For this review, take the finished solid that the model builds, in its own axes (mm). A direction names the side the tool comes from. Round coordinates to 2 decimals unless told otherwise and drop trailing zeros. Order: outer loops, then holes, each group sorted by start corner. A loop starts at its lowest first (then second) coordinate and runs counter-clockwise, first axis right, second up. Notation, with made-up numbers: M 14.25,50.5 L 24.25,50.5 A31 cw 24.25,74.5 Z; hole C -28,73 d8. An arc over 180 degrees is marked long. Answer as a JSON object with one key per item and string values.
from build123d import *

# Parameters (mm, degrees)
SKETCH1_W                        = 203.2
SKETCH1_H                        = 50.8
BOSS_EXTRUDE1_DEPTH              = 1
SKETCH1_3_R                      = 6.477
BOSS_EXTRUDE2_DEPTH              = 2.54
SKETCH2_W                        = 4.9022
SKETCH2_H                        = 3.54
F_3_8_CLEARANCE_HOLE1_AT_2_COUNT = 2
F_3_8_CLEARANCE_HOLE1_AT_2_PITCH = 69.85
F_3_8_CLEARANCE_HOLE1_AT_3_COUNT = 2
F_3_8_CLEARANCE_HOLE1_AT_3_PITCH = 139.7
F_3_8_CLEARANCE_HOLE1_AT_4_COUNT = 2
F_3_8_CLEARANCE_HOLE1_AT_4_PITCH = 69.85
FILLET1_R                        = 12.7


with BuildPart() as part:
    # Sketch1 → Boss-Extrude1 (new body)
    with BuildSketch(Plane.XY):
        with Locations((-9.525, 0)):
            Rectangle(SKETCH1_W, SKETCH1_H)
    extrude(amount=BOSS_EXTRUDE1_DEPTH)

    # Sketch1<3> → Boss-Extrude2 (add)
    with BuildSketch(Plane.XY):
        with Locations((-69.85, 0)):
            Circle(SKETCH1_3_R)
        Circle(SKETCH1_3_R)
        with Locations((69.85, 0)):
            Circle(SKETCH1_3_R)
    extrude(amount=-BOSS_EXTRUDE2_DEPTH)

    # Sketch2 → 3/8 Clearance Hole1 (revolve, cut)
    with BuildSketch(Plane(origin=(-69.85, 0, 1), x_dir=(0, -1, 0), z_dir=(1, 0, 0))):
        with Locations((2.4511, 1.77)):
            Rectangle(SKETCH2_W, SKETCH2_H)
    f_3_8_clearance_hole1 = revolve(axis=Axis((-69.85, 0, 7.35), (0, 0, -1)), mode=Mode.SUBTRACT)

    # 3/8 Clearance Hole1 at 2: 3/8 Clearance Hole1 ×2
    with Locations(*[(i * F_3_8_CLEARANCE_HOLE1_AT_2_PITCH, 0, 0) for i in range(1, F_3_8_CLEARANCE_HOLE1_AT_2_COUNT)]):
        add(f_3_8_clearance_hole1, mode=Mode.SUBTRACT)

    # 3/8 Clearance Hole1 at 3: 3/8 Clearance Hole1 ×2
    with Locations(*[(i * F_3_8_CLEARANCE_HOLE1_AT_3_PITCH, 0, 0) for i in range(1, F_3_8_CLEARANCE_HOLE1_AT_3_COUNT)]):
        add(f_3_8_clearance_hole1, mode=Mode.SUBTRACT)

    # 3/8 Clearance Hole1 at 4: 3/8 Clearance Hole1 ×2
    with Locations(*[(i * F_3_8_CLEARANCE_HOLE1_AT_4_PITCH, 0, 0) for i in range(1, F_3_8_CLEARANCE_HOLE1_AT_4_COUNT)]):
        add(f_3_8_clearance_hole1, mode=Mode.SUBTRACT)

    # Fillet1
    fillet1_edges = [part.edges().sort_by_distance(p)[0] for p in [
        (92.075, -25.4, 0.5),
        (-111.125, -25.4, 0.5),
        (-111.125, 25.4, 0.5),
        (92.075, 25.4, 0.5),
    ]]
    fillet(fillet1_edges, radius=FILLET1_R)


solid = part.part
1) Add section D-D on x = -87.5. State the section outline as (y, z) points, and give its area (3 significant figures).
Geometry check:
{"outline": "M -25.4,0 L 25.4,0 L 25.4,1 L -25.4,1 Z", "area": "50.8 mm²"}
2) Machinability: for faces 4 (the flat face through (-1, 5, -2.54)), 5 (the cylindrical face through (63.38, 0.28, -1.25)), which of the approach directions +Z, -Z, +X, -X, +Y, -Y give a long, thin tool a straight path to every point of the face, cutting with its end or side? Answer none if there is none.
Geometry check:
{"face 4": "-Z, +X, -X, +Y, -Y", "face 5": "-Z"}
3) Add section B-B on x = 0. State the section outline as (y, z) points.
Geometry check:
{"outline": "M -25.4,0 L -6.48,0 L -6.48,-2.54 L -4.9,-2.54 L -4.9,1 L -25.4,1 Z; M 4.9,-2.54 L 6.48,-2.54 L 6.48,0 L 25.4,0 L 25.4,1 L 4.9,1 Z"}
4) Add section A-A on z = -1.55. State the section outline as (x, y) points.
Geometry check:
{"outline": "C -69.85,0 d12.95; C 0,0 d12.95; C 69.85,0 d12.95; hole C -69.85,0 d9.8; hole C 0,0 d9.8; hole C 69.85,0 d9.8"}
5) Insertion check: P1, Ø1.5, axis at x = -71.5, z = -1, coming from the +Y side; P2, Ø1, axis at x = 38.5, y = 8.5, coming from the -Z side. Each pin has a flat end and moves straight along its axis. Give the tip position at first contact, or say it passes through.
Geometry check:
{"P1": "stops at y = 6.41", "P2": "stops at z = 0"}
6) Add section C-C on y = 0. State the section outline as (x, z) points (3 decimals), and give its area (3 significant figures).
Geometry check:
{"outline": "M -111.125,0 L -76.327,0 L -76.327,-2.54 L -74.752,-2.54 L -74.752,1 L -111.125,1 Z; M -64.948,-2.54 L -63.373,-2.54 L -63.373,0 L -6.477,0 L -6.477,-2.54 L -4.902,-2.54 L -4.902,1 L -64.948,1 Z; M 4.902,-2.54 L 6.477,-2.54 L 6.477,0 L 63.373,0 L 63.373,-2.54 L 64.948,-2.54 L 64.948,1 L 4.902,1 Z; M 74.752,-2.54 L 76.327,-2.54 L 76.327,0 L 92.075,0 L 92.075,1 L 74.752,1 Z", "area": "198 mm²"}
7) For L1, parallel to X at y = 0, z = 0.35 (3 decimals); L2, parallel to Y at x = -69.85, z = -1.25; L3, parallel to X at y = 1, z = -1.4, list the stretches that pass through material, from the lowest coordinate up.
Geometry check:
{"L1": "x = -111.125 to -74.752, -64.948 to -4.902, 4.902 to 64.948, 74.752 to 92.075", "L2": "y = -6.48 to -4.9, 4.9 to 6.48", "L3": "x = -76.25 to -74.65, -65.05 to -63.45, -6.4 to -4.8, 4.8 to 6.4, 63.45 to 65.05, 74.65 to 76.25"}
8) Mouldability with a two-part tool opening along X and no side actions: class faces 1 (the cylindrical face through (-3.313, 3.613, -0.795)), 2 (the cylindrical face through (88.256, 21.778, 0.507)), 3 (the flat face through (69, 5, -2.54)) as +X half, -X half, draft (parallel to the pull), parting line (faces both ways), or undercut.
Geometry check:
{"face 1": "undercut", "face 2": "+X half", "face 3": "draft"}
